For this review, take the finished solid that the model builds, in its own axes (mm). A direction names the side the tool comes from. Give positions to 0.01 mm unless a question says otherwise; leave off trailing zeros. Order: outer loops, then holes, each group sorted by start corner. A loop starts at its lowest first (then second) coordinate and runs counter-clockwise, first axis right, second up. Notation, with made-up numbers: (55.25, -11) - (110.25, -11) arc R23 ccw to (110.25, 15) - close; hole circle Ø7 at (56.25, 33.5). An arc over 180 degrees is marked (long way). One line per item, written item: value.
```python
from build123d import *

# Parameters (mm, degrees)
F1_DEPTH = 76.2
F4_DEPTH = 50.8
F7_D     = 2.54
F6_W     = 12.7
F6_H     = 88.9
F8_DEPTH = 6.35
F9_R     = 5.08
F10_R    = 3.17499


# Not quite as in the source:
# - a fillet or chamfer is up to 0.001 mm smaller than in the source, because OpenCascade refuses the exact size


with BuildPart() as f1:
    # F0 (on Front) → F1 (new body)
    with BuildSketch(Plane.XZ):
        with BuildLine():
            Line((-74.9020473927, -80.410034281), (-74.9020473927, -83.585034281))
            Line((-74.9020473927, -83.585034281), (77.4979526073, -83.585034281))
            Line((77.4979526073, -83.585034281), (77.4979526073, -77.235034281))
            Line((77.4979526073, -77.235034281), (77.4979526073, 11.664965719))
            Line((77.4979526073, 11.664965719), (71.1479526073, 11.664965719))
            Line((71.1479526073, 11.664965719), (71.1479526073, -77.235034281))
            Line((71.1479526073, -77.235034281), (17.9289044716, -77.235034281))
            ThreePointArc((17.9289044716, -77.235034281), (13.4387764111, -75.3751623415), (11.5789044716, -70.885034281))
            Line((11.5789044716, -70.885034281), (11.5789044716, 46.589965719))
            ThreePointArc((11.5789044716, 46.589965719), (10.6489685019, 48.8350297493), (8.4039044716, 49.764965719))
            Line((8.4039044716, 49.764965719), (-23.3460955284, 49.764965719))
            ThreePointArc((-23.3460955284, 49.764965719), (-25.5911595586, 48.8350297493), (-26.5210955284, 46.589965719))
            Line((-26.5210955284, 46.589965719), (-26.5210955284, -70.885034281))
            ThreePointArc((-26.5210955284, -70.885034281), (-28.3809674678, -75.3751623415), (-32.8710955284, -77.235034281))
            Line((-32.8710955284, -77.235034281), (-71.7270473927, -77.235034281))
            ThreePointArc((-71.7270473927, -77.235034281), (-73.972111423, -78.1649702507), (-74.9020473927, -80.410034281))
        make_face()
        with BuildLine():
            ThreePointArc((-9.0585955284, -3.784664938), (-10.6460955284, -1.035034281), (-9.0585955284, 1.714596376))
            Line((-9.0585955284, 1.714596376), (-9.0585955284, 3.553124576))
            Line((-9.0585955284, 3.553124576), (-5.8835955284, 3.553124576))
            Line((-5.8835955284, 3.553124576), (-5.8835955284, 1.714596376))
            ThreePointArc((-5.8835955284, 1.714596376), (-4.2960955284, -1.035034281), (-5.8835955284, -3.784664938))
            Line((-5.8835955284, -3.784664938), (-5.8835955284, -5.623193138))
            Line((-5.8835955284, -5.623193138), (-9.0585955284, -5.623193138))
            Line((-9.0585955284, -5.623193138), (-9.0585955284, -3.784664938))
        make_face(mode=Mode.SUBTRACT)
    extrude(amount=F1_DEPTH)

    # F3 (on offset) → F4 (cut, through all)
    with BuildSketch(Plane(origin=(0, -12.7, 0), x_dir=(-1, 0, 0), z_dir=(0, 1, 0))):
        with BuildLine():
            Line((-17.9289044716, -77.235034281), (32.8710955284, -77.235034281))
            ThreePointArc((32.8710955284, -77.235034281), (28.3809674678, -75.3751623415), (26.5210955284, -70.885034281))
            Line((26.5210955284, -70.885034281), (26.5210955284, 46.589965719))
            ThreePointArc((26.5210955284, 46.589965719), (25.5911595586, 48.8350297493), (23.3460955284, 49.764965719))
            Line((23.3460955284, 49.764965719), (-8.4039044716, 49.764965719))
            ThreePointArc((-8.4039044716, 49.764965719), (-10.6489685019, 48.8350297493), (-11.5789044716, 46.589965719))
            Line((-11.5789044716, 46.589965719), (-11.5789044716, -70.885034281))
            ThreePointArc((-11.5789044716, -70.885034281), (-13.4387764111, -75.3751623415), (-17.9289044716, -77.235034281))
        make_face()
    extrude(amount=-F4_DEPTH, mode=Mode.SUBTRACT)

    # F7 (through all)
    with Locations(Plane.YZ.offset(77.4979526073)):
        with Locations((-44.846875, -9.3153121099), (-31.353125, -9.3153121099)):
            Hole(F7_D / 2)

    # F6 (on offset) → F8 (cut)
    with BuildSketch(Plane.YZ.offset(77.4979526073)):
        with Locations((-69.85, -32.785034281)):
            Rectangle(F6_W, F6_H)
        with Locations((-6.35, -32.785034281)):
            Rectangle(F6_W, F6_H)
    extrude(amount=-F8_DEPTH, mode=Mode.SUBTRACT)

    # F9
    f9_edges = [f1.edges().sort_by_distance(p)[0] for p in [
        (74.322953, -12.7, -77.235034),
        (71.147953, -38.1, -77.235034),
        (74.322953, -63.5, -77.235034),
    ]]
    fillet(f9_edges, radius=F9_R)

    # F10 (radius 3.175 in the source; OpenCascade refuses exactly that, so slightly less here)
    f10_edges = [f1.edges().sort_by_distance(p)[0] for p in [
        (74.322953, -63.5, 11.664966),
        (74.322953, -12.7, 11.664966),
        (77.497953, -38.1, 11.664966),
        (71.147953, -38.1, 11.664966),
    ]]
    fillet(f10_edges, radius=F10_R)


solid = f1.part
```
(1) Take a section at A-A (z = 36). Write out the cut boundary in (x, y).
Answers below:
outline: (-26.52, -76.2) - (11.58, -76.2) - (11.58, -63.5) - (-26.52, -63.5) - close; (-26.52, -12.7) - (11.58, -12.7) - (11.58, 0) - (-26.52, 0) - close
(2) Take a section at B-B (z = -23). Write out the cut boundary in (x, y), then the cut area to 3 significant figures.
Answers below:
outline: (-26.52, -76.2) - (11.58, -76.2) - (11.58, -63.5) - (-26.52, -63.5) - close; (-26.52, -12.7) - (11.58, -12.7) - (11.58, 0) - (-26.52, 0) - close; (71.15, -63.5) - (77.5, -63.5) - (77.5, -12.7) - (71.15, -12.7) - close
area: 1,290 mm^2
(3) Take a section at D-D (z = -1). Write out the cut boundary in (x, y), then the cut area to 3 significant figures.
Answers below:
outline: (-26.52, -76.2) - (-10.65, -76.2) - (-10.65, -63.5) - (-26.52, -63.5) - close; (-26.52, -12.7) - (-10.65, -12.7) - (-10.65, 0) - (-26.52, 0) - close; (-4.3, -76.2) - (11.58, -76.2) - (11.58, -63.5) - (-4.3, -63.5) - close; (-4.3, -12.7) - (11.58, -12.7) - (11.58, 0) - (-4.3, 0) - close; (71.15, -63.5) - (77.5, -63.5) - (77.5, -12.7) - (71.15, -12.7) - close
area: 1,130 mm^2
(4) Machinability: for faces 1 (the face through (-10.646, -6.261, -1.082)), 2 (the face through (74, -63.5, -32)), 3 (the face through (11.579, -70, -13)), 4 (the face through (4, -38, -77.235)), which of the approach directions +Z, -Z, +X, -X, +Y, -Y give a long, thin tool a straight path to every point of the face, cutting with its end or side? Answer none if there is none.
Answers below:
face 1: +Y, -Y
face 2: +Z, +X, -Y
face 3: +Z, +X, +Y, -Y
face 4: +Z
(5) Draft analysis for pull direction Z (two halves, no side actions). For faces 5 (the face through (-5, 0, -22)), 6 (the face through (-28.332, -69.761, -75.326)), 7 (the face through (-4.296, -69.761, -0.988)), state which applies: pulls with the +Z half, pulls with the -Z half, needs draft (parallel to the pull), parting line crosses it, or undercut.
Answers below:
face 5: needs draft
face 6: pulls with the +Z half
face 7: undercut
(6) Wall thickness on line 1 (Y direction, x = -22.5, z = -61.5); line 2 (Z direction, x = -62, y = -57.5); line 3 (X direction, y = -59, z = -1): over which ranges is each line inside the solid? List them lowest first. Write a range as from..to.
Answers below:
line 1: y = -76.2..-63.5, -12.7..0
line 2: z = -83.59..-77.24
line 3: x = 71.15..77.5
(7) For P1, Ø14, axis at y = -8.5, z = -13.5, coming from the -X side; P2, Ø4, axis at y = -44.85, z = -9.32, coming from the -X side; P3, Ø6, axis at x = 18, y = -32.5, coming from the +Z side, all flat-tipped, find the tip position at first contact; note any pin that passes through.
Answers below:
P1: stops at x = -26.52
P2: stops at x = 71.15
P3: stops at z = -77.24
